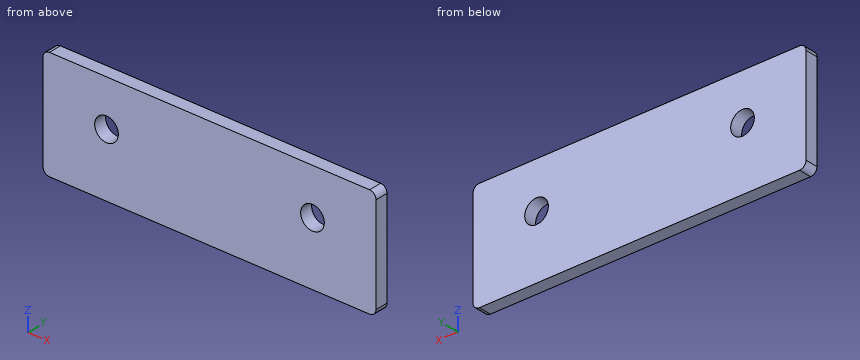
from build123d import *

# Parameters (mm, degrees)
F0_W     = 327.289753
F0_H     = 107.929777
F0_R     = 11.624246
F1_DEPTH = 12.7
F2_R     = 6.35


with BuildPart() as f1:
    # F0 (on Front) → F1 (new body)
    with BuildSketch(Plane.XZ):
        with Locations((20.452689, 12.309231)):
            Rectangle(F0_W, F0_H)
        with Locations((-80.767942, 20.768589)):
            Circle(F0_R, mode=Mode.SUBTRACT)
        with Locations((121.673319, 20.768589)):
            Circle(F0_R, mode=Mode.SUBTRACT)
    extrude(amount=F1_DEPTH)

    # F2
    f2_edges = [f1.edges().sort_by_distance(p)[0] for p in [
        (-143.192188, -6.35, 66.27412),
        (-143.192188, -6.35, -41.655657),
        (184.097565, -6.35, -41.655657),
        (184.097565, -6.35, 66.27412),
    ]]
    fillet(f2_edges, radius=F2_R)


solid = f1.part
Source: CAD feature listing. Evaluate the final solid. Frame: model axes, mm. Give positions to 0.01 mm unless a question says otherwise; leave off trailing zeros. Write each loop counter-clockwise with the first axis right and the second up, starting at its lowest first coordinate (ties: lowest second). Pieces come first, ordered by that corner, then holes. Notation, with made-up numbers: (66.5, 6.25) -> (121.5, 6.25) arc R17 ccw to (121.5, 38.25) -> close; hole circle Ø9 at (48, -14). An arc over 180 degrees is marked (long way). Return JSON: item names as keys, results as strings. Group by question number.
1. Section A-A, the plane z = 18. Output: boundary loops of the cut face in (x, y), then the cut area to 3 significant figures.
2. Material intervals for line 1 (X direction, y = -10.5, z = 29.5); line 2 (X direction, y = -8.5, z = 25.5); line 3 (Z direction, x = -74, y = -7.25), sorted ascending. Write a range as from..to.
3. Section B-B, the plane x = -89.5. Output: boundary loops of the cut face in (y, z), then the cut area to 3 significant figures.
4. Section C-C, the plane y = -9.5. Output: boundary loops of the cut face in (x, z), then the cut area to 3 significant figures.
Determined:
{
 "1": {"outline": "(-143.19, -12.7) -> (-92.06, -12.7) -> (-92.06, 0) -> (-143.19, 0) -> close; (-69.48, -12.7) -> (110.38, -12.7) -> (110.38, 0) -> (-69.48, 0) -> close; (132.96, -12.7) -> (184.1, -12.7) -> (184.1, 0) -> (132.96, 0) -> close", "area": "3,580 mm2"},
 "2": {"line 1": "x = -143.19..-88.44, -73.09..114, 129.35..184.1", "line 2": "x = -143.19..-91.39, -70.15..111.06, 132.29..184.1", "line 3": "z = -41.66..11.32, 30.22..66.27"},
 "3": {"outline": "(-12.7, -41.66) -> (0, -41.66) -> (0, 13.1) -> (-12.7, 13.1) -> close; (-12.7, 28.44) -> (0, 28.44) -> (0, 66.27) -> (-12.7, 66.27) -> close", "area": "1,180 mm2"},
 "4": {"outline": "(-143.19, -35.31) arc R6.35 ccw to (-136.84, -41.66) -> (177.75, -41.66) arc R6.35 ccw to (184.1, -35.31) -> (184.1, 59.92) arc R6.35 ccw to (177.75, 66.27) -> (-136.84, 66.27) arc R6.35 ccw to (-143.19, 59.92) -> close; hole circle Ø23.25 at (-80.77, 20.77); hole circle Ø23.25 at (121.67, 20.77)", "area": "34,400 mm2"}
}
